Here's how the part is built. I have some questions about the finished solid (model axes, mm). A direction names the side the tool comes from. Coordinates: 2 decimals unless noted, no trailing zeros. Loops run counter-clockwise (first coordinate to the right, second up) from the corner with the lowest first, then second, coordinate; pieces in that order, holes last. Notation, with made-up numbers: (38.5, -2.75) -> (50.5, -2.75) arc R31 ccw to (50.5, 23.25) -> close; hole circle Ø3 at (9.25, 46). An arc over 180 degrees is marked (long way). Answer as a JSON object with one key per item and string values. Group by question number.
Q1. I'm going to push a flat-ended pin straight in: pin 1 (2 mm diameter, centred on y = -12, z = 2, fed in from +X). Where does the tip first touch, or does it pass through?
Q2. Thinking about a two-plate mould opening in X: for faces 4 (the flat face through (-69, -10, 2)), 5 (the flat face through (-72, -24, 2)), 6 (the flat face through (-2, 50, 2)), which applies, released by +X, released by -X, zero draft, split by the parting line, or undercut?
Q3. I need wall thicknesses on line 1 (Y direction, x = -44, z = 2.65); line 2 (X direction, y = 42.5, z = 3.15); line 3 (X direction, y = -40.5, z = 1.4). Which ranges of each line are inside material? Lowest first, please.
Q4. On a 3-axis mill with a long thin cutter (end or side, diameter ignored), from which of +Z, -Z, +X, -X, +Y, -Y can I reach the whole of each face in a straight line? I mean faces 1 (the flat face through (-69, 42, 2)), 2 (the flat face through (-72, 32, 2)), 3 (the flat face through (-56, -21, 2)). Say none if no direction works.
Q5. I want a section at A-A on x = -44. Write out the boundary of the cut face in (y, z).
Q6. I want a section at B-B on z = 1.05. Count the separate pieces of the cut face and the enclosed holes in it, then the cut area to 3 significant figures.
```python
from build123d import *

# Parameters (mm, degrees)
SKETCH1_W           = 144
SKETCH1_H           = 115
SKETCH1_R           = 3.5
SKETCH1_W_2         = 4
SKETCH1_H_2         = 4
BOSS_EXTRUDE1_DEPTH = 4
SKETCH2_W           = 6
SKETCH2_H           = 4
CUT_EXTRUDE1_DEPTH  = 4
SKETCH4_W           = 4
SKETCH4_H           = 4
CUT_EXTRUDE2_DEPTH  = 10


with BuildPart() as part:
    # Sketch1 → Boss-Extrude1 (new body)
    with BuildSketch(Plane.XY):
        Rectangle(SKETCH1_W, SKETCH1_H)
        with Locations((-44, 37)):
            Circle(SKETCH1_R, mode=Mode.SUBTRACT)
        with Locations((44, 37)):
            Circle(SKETCH1_R, mode=Mode.SUBTRACT)
        with Locations((44, -23)):
            Circle(SKETCH1_R, mode=Mode.SUBTRACT)
        with Locations((-44, -23)):
            Circle(SKETCH1_R, mode=Mode.SUBTRACT)
        with Locations((0, 42)):
            Rectangle(SKETCH1_W_2, SKETCH1_H_2, mode=Mode.SUBTRACT)
        with BuildLine():
            Line((-24, 27), (24, 27))
            ThreePointArc((24, 27), (31.071067812, 24.071067812), (34, 17))
            Line((34, 17), (34, -3))
            ThreePointArc((34, -3), (31.071067812, -10.071067812), (24, -13))
            Line((24, -13), (-24, -13))
            ThreePointArc((-24, -13), (-31.071067812, -10.071067812), (-34, -3))
            Line((-34, -3), (-34, 17))
            ThreePointArc((-34, 17), (-31.071067812, 24.071067812), (-24, 27))
        make_face(mode=Mode.SUBTRACT)
        with Locations((0, 50)):
            Rectangle(SKETCH1_W_2, SKETCH1_H_2, mode=Mode.SUBTRACT)
        with Locations((0, 34)):
            Rectangle(SKETCH1_W_2, SKETCH1_H_2, mode=Mode.SUBTRACT)
        with Locations((0, -34)):
            Rectangle(SKETCH1_W_2, SKETCH1_H_2, mode=Mode.SUBTRACT)
        with Locations((0, -42)):
            Rectangle(SKETCH1_W_2, SKETCH1_H_2, mode=Mode.SUBTRACT)
        with Locations((0, -50)):
            Rectangle(SKETCH1_W_2, SKETCH1_H_2, mode=Mode.SUBTRACT)
    extrude(amount=BOSS_EXTRUDE1_DEPTH)

    # Sketch2 → Cut-Extrude1 (cut)
    with BuildSketch(Plane.XY.offset(4)):
        with Locations((-69, 12)):
            Rectangle(SKETCH2_W, SKETCH2_H)
        with Locations((-69, 4)):
            Rectangle(SKETCH2_W, SKETCH2_H)
        with Locations((-69, 20)):
            Rectangle(SKETCH2_W, SKETCH2_H)
        with Locations((-69, 28)):
            Rectangle(SKETCH2_W, SKETCH2_H)
        with Locations((-69, 36)):
            Rectangle(SKETCH2_W, SKETCH2_H)
        with Locations((-69, 44)):
            Rectangle(SKETCH2_W, SKETCH2_H)
        with Locations((69, 44)):
            Rectangle(SKETCH2_W, SKETCH2_H)
        with Locations((69, 36)):
            Rectangle(SKETCH2_W, SKETCH2_H)
        with Locations((69, 28)):
            Rectangle(SKETCH2_W, SKETCH2_H)
        with Locations((69, 20)):
            Rectangle(SKETCH2_W, SKETCH2_H)
        with Locations((69, 4)):
            Rectangle(SKETCH2_W, SKETCH2_H)
        with Locations((69, 12)):
            Rectangle(SKETCH2_W, SKETCH2_H)
        with Locations((69, -12)):
            Rectangle(SKETCH2_W, SKETCH2_H)
        with Locations((69, -4)):
            Rectangle(SKETCH2_W, SKETCH2_H)
        with Locations((69, -20)):
            Rectangle(SKETCH2_W, SKETCH2_H)
        with Locations((69, -28)):
            Rectangle(SKETCH2_W, SKETCH2_H)
        with Locations((69, -36)):
            Rectangle(SKETCH2_W, SKETCH2_H)
        with Locations((69, -44)):
            Rectangle(SKETCH2_W, SKETCH2_H)
        with Locations((-69, -44)):
            Rectangle(SKETCH2_W, SKETCH2_H)
        with Locations((-69, -36)):
            Rectangle(SKETCH2_W, SKETCH2_H)
        with Locations((-69, -28)):
            Rectangle(SKETCH2_W, SKETCH2_H)
        with Locations((-69, -20)):
            Rectangle(SKETCH2_W, SKETCH2_H)
        with Locations((-69, -4)):
            Rectangle(SKETCH2_W, SKETCH2_H)
        with Locations((-69, -12)):
            Rectangle(SKETCH2_W, SKETCH2_H)
    extrude(amount=-CUT_EXTRUDE1_DEPTH, mode=Mode.SUBTRACT)

    # Sketch4 → Cut-Extrude2 (cut)
    with BuildSketch(Plane.XY.offset(4)):
        with Locations((8, -19)):
            Rectangle(SKETCH4_W, SKETCH4_H)
        with Locations((16, -19)):
            Rectangle(SKETCH4_W, SKETCH4_H)
        with Locations((24, -19)):
            Rectangle(SKETCH4_W, SKETCH4_H)
        with Locations((32, -19)):
            Rectangle(SKETCH4_W, SKETCH4_H)
        with Locations((56, -19)):
            Rectangle(SKETCH4_W, SKETCH4_H)
        with Locations((-56, -19)):
            Rectangle(SKETCH4_W, SKETCH4_H)
        with Locations((-32, -19)):
            Rectangle(SKETCH4_W, SKETCH4_H)
        with Locations((-24, -19)):
            Rectangle(SKETCH4_W, SKETCH4_H)
        with Locations((-16, -19)):
            Rectangle(SKETCH4_W, SKETCH4_H)
        with Locations((-8, -19)):
            Rectangle(SKETCH4_W, SKETCH4_H)
        with Locations((8, 33)):
            Rectangle(SKETCH4_W, SKETCH4_H)
        with Locations((16, 33)):
            Rectangle(SKETCH4_W, SKETCH4_H)
        with Locations((24, 33)):
            Rectangle(SKETCH4_W, SKETCH4_H)
        with Locations((32, 33)):
            Rectangle(SKETCH4_W, SKETCH4_H)
        with Locations((-56, 33)):
            Rectangle(SKETCH4_W, SKETCH4_H)
        with Locations((-32, 33)):
            Rectangle(SKETCH4_W, SKETCH4_H)
        with Locations((56, 33)):
            Rectangle(SKETCH4_W, SKETCH4_H)
        with Locations((-24, 33)):
            Rectangle(SKETCH4_W, SKETCH4_H)
        with Locations((-16, 33)):
            Rectangle(SKETCH4_W, SKETCH4_H)
        with Locations((-8, 33)):
            Rectangle(SKETCH4_W, SKETCH4_H)
    extrude(amount=-CUT_EXTRUDE2_DEPTH, mode=Mode.SUBTRACT)


solid = part.part
```
Result set:
{
 "1": {"pin 1": "stops at x = 66"},
 "2": {"face 4": "zero draft", "face 5": "released by -X", "face 6": "undercut"},
 "3": {"line 1": "y = -57.5 to -26.5, -19.5 to 33.5, 40.5 to 57.5", "line 2": "x = -66 to -2, 2 to 66", "line 3": "x = -72 to -2, 2 to 72"},
 "4": {"face 1": "+Z, -Z, -X", "face 2": "+Z, -Z, -X, +Y, -Y", "face 3": "+Z, -Z"},
 "5": {"outline": "(-57.5, 0) -> (-26.5, 0) -> (-26.5, 4) -> (-57.5, 4) -> close; (-19.5, 0) -> (33.5, 0) -> (33.5, 4) -> (-19.5, 4) -> close; (40.5, 0) -> (57.5, 0) -> (57.5, 4) -> (40.5, 4) -> close"},
 "6": {"separate pieces": "1", "enclosed holes": "31", "area": "12,800 mm²"}
}
